Can you work these out from the model? Positions are in its coordinate system, mm. Round coordinates to 2 decimals unless told otherwise and drop trailing zeros. Order: outer loops, then holes, each group sorted by start corner. A loop starts at its lowest first (then second) coordinate and runs counter-clockwise, first axis right, second up. Notation, with made-up numbers: (50.25, 36.5) - (76.25, 36.5) arc R15 cw to (76.25, 56.5) - close; hole circle Ø3 at (36, -29.5). An arc over 180 degrees is marked (long way). Write item = value, one per line.
from build123d import *

# Parameters (mm, degrees)
F1_DEPTH = 2
F5_DEPTH = 25
F6_DEPTH = 2


with BuildPart() as f1:
    # F0 (on Top) → F1 (new body)
    with BuildSketch(Plane.XY):
        with BuildLine():
            Line((-0.002053, 3.432452), (-2.304997, 5.735396))
            ThreePointArc((-2.304997, 5.735396), (-5.69911, 5.735396), (-5.69911, 2.341283))
            Line((-5.69911, 2.341283), (-3.396166, 0.038339))
            Line((-3.396166, 0.038339), (-5.69911, -2.264604))
            ThreePointArc((-5.69911, -2.264604), (-5.69911, -5.658717), (-2.304997, -5.658717))
            Line((-2.304997, -5.658717), (-0.002053, -3.355773))
            Line((-0.002053, -3.355773), (2.30089, -5.658717))
            ThreePointArc((2.30089, -5.658717), (5.695003, -5.658717), (5.695003, -2.264604))
            Line((5.695003, -2.264604), (3.392059, 0.038339))
            Line((3.392059, 0.038339), (5.695003, 2.341283))
            ThreePointArc((5.695003, 2.341283), (5.695003, 5.735396), (2.30089, 5.735396))
            Line((2.30089, 5.735396), (-0.002053, 3.432452))
        make_face()
    extrude(amount=F1_DEPTH)



with BuildPart() as f3:
    # F2 (on Front) → F3 (revolve)
    with BuildSketch(Plane.XZ):
        with BuildLine():
            Line((24.997947, 1), (-25.002053, 1))
            ThreePointArc((-25.002053, 1), (-0.002053, -24), (24.997947, 1))
        make_face()
    revolve(axis=Axis((-0.456872, 0, 1), (1, 0, 0)))

    # F4 (on Top) → F5 (cut)
    with BuildSketch(Plane.XY):
        with BuildLine():
            Line((12.997947, 16), (-13.002053, 16))
            ThreePointArc((-13.002053, 16), (-15.123374, 15.12132), (-16.002053, 13))
            Line((-16.002053, 13), (-16.002053, -13))
            ThreePointArc((-16.002053, -13), (-15.123374, -15.12132), (-13.002053, -16))
            Line((-13.002053, -16), (12.997947, -16))
            ThreePointArc((12.997947, -16), (15.119267, -15.12132), (15.997947, -13))
            Line((15.997947, -13), (15.997947, 13))
            ThreePointArc((15.997947, 13), (15.119267, 15.12132), (12.997947, 16))
        make_face()
    extrude(amount=-F5_DEPTH, mode=Mode.SUBTRACT)


with BuildPart() as f1_1:
    add(f1.part)

    add(f3.part)  # F6 merges F3
    # F0 (on Top) → F6 (join)
    with BuildSketch(Plane.XY):
        with BuildLine():
            Line((-0.002053, 3.432452), (-2.304997, 5.735396))
            ThreePointArc((-2.304997, 5.735396), (-5.69911, 5.735396), (-5.69911, 2.341283))
            Line((-5.69911, 2.341283), (-3.396166, 0.038339))
            Line((-3.396166, 0.038339), (-5.69911, -2.264604))
            ThreePointArc((-5.69911, -2.264604), (-5.69911, -5.658717), (-2.304997, -5.658717))
            Line((-2.304997, -5.658717), (-0.002053, -3.355773))
            Line((-0.002053, -3.355773), (2.30089, -5.658717))
            ThreePointArc((2.30089, -5.658717), (5.695003, -5.658717), (5.695003, -2.264604))
            Line((5.695003, -2.264604), (3.392059, 0.038339))
            Line((3.392059, 0.038339), (5.695003, 2.341283))
            ThreePointArc((5.695003, 2.341283), (5.695003, 5.735396), (2.30089, 5.735396))
            Line((2.30089, 5.735396), (-0.002053, 3.432452))
        make_face()
    extrude(amount=-F6_DEPTH)


solid = f1_1.part
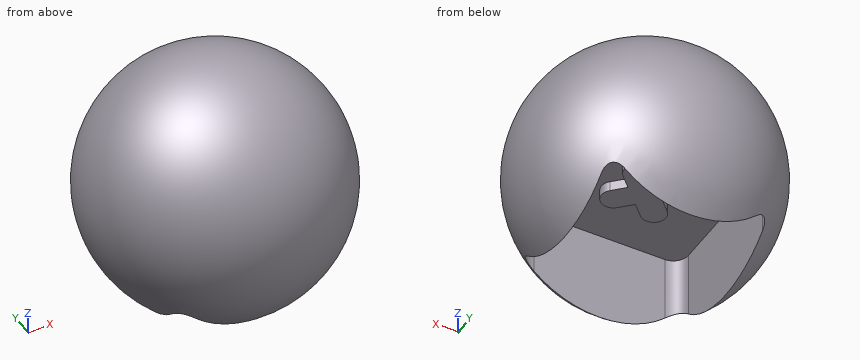
(1) If we section it at A-A (z = -10): Write out the boundary of the cut face in (x, y).
Computed:
outline = circle Ø44.9 at (0, 0); hole (-16, -13) arc R3 ccw to (-13, -16) - (13, -16) arc R3 ccw to (16, -13) - (16, 13) arc R3 ccw to (13, 16) - (-13, 16) arc R3 ccw to (-16, 13) - close
(2) Will these pins go through, and if not, where does the flat tip stop? P1, Ø5, axis at x = -17.5, z = 10.5, coming from the +Y side; P2, Ø1.5, axis at y = -11, z = 16.5, coming from the +X side; P3, Ø5, axis at x = 1.5, y = 13, coming from the -Z side.
Computed:
P1 = 17.94
P2 = 17.08
P3 = 0
(3) If we section it at B-B (x = -5): Write out the boundary of the cut face in (y, z).
Computed:
outline = (-16, -17.55) - (-16, 0) - (-6.14, 0) - (-6.14, -2) - (-1.57, -2) - (-1.57, 0) - (1.64, 0) - (1.64, -2) - (6.22, -2) - (6.22, 0) - (16, 0) - (16, -17.55) arc R24.5 ccw (long way) to start
(4) If we section it at C-C (y = 12): Write out the boundary of the cut face in (x, z), plus the area to 3 significant figures.
Computed:
outline = (-16, -14) - (-16, 0) - (16, 0) - (16, -14) arc R21.93 ccw (long way) to start
area = 910 mm^2
(5) If we section it at D-D (z = 20.5): Write out the boundary of the cut face in (x, y).
Computed:
outline = circle Ø31.29 at (0, 0)
(6) If I drill on line 1 (Y direction, x = -5, z = -0.5); line 2 (Y direction, x = -3, z = -6.5); line 3 (X direction, y = -7, z = -2), over which ranges is the centre line in solid material (lowest first)? Write a range as from..to.
Computed:
line_1 = -24.45..-16, -6.14..-1.57, 1.64..6.22, 16..24.45
line_2 = -23.66..-16, 16..23.66
line_3 = -23.81..-16, 16..23.81
